Model file for the job. Use its own axes, mm. Face numbers are marked on the shaded views. Coordinates: 2 decimals unless noted, no trailing zeros. Write each loop counter-clockwise with the first axis right and the second up, starting at its lowest first coordinate (ties: lowest second). Pieces come first, ordered by that corner, then holes. Notation, with made-up numbers: (23.5, -12) - (75.5, -12) arc R23 ccw to (75.5, 11) - close; hole circle Ø5 at (41.25, 24). An arc over 180 degrees is marked (long way). Put each result on its own line as item: value. Start each with the question number.
1. Saw through at B-B, the plane z = -3.1. Write the cut outline in (x, y).
2. Drill centre lines: L1, parallel to Y at x = 686.5, z = -1.85; L2, parallel to Z at x = 697, y = -1297; L3, parallel to X at y = -1252, z = -1.25. Where is each one in solid material? Low to high. Write a range as from..to.
3. Drop flat-ended pins along their axis: P1, Ø2, axis at y = -1269.5, z = -2.5, coming from the +X side; P2, Ø4, axis at x = 681, y = -1314, coming from the -Z side. Give the stop position or say it passes through.
4. Saw through at A-A, the plane x = 663. Write the cut outline in (y, z).
5. Pull direction Y, two halves, no side cores. Call the marked faces 1 and 2: released by +Y, released by -Y, zero draft, split by the parting line, or undercut.
6. Saw through at C-C, the plane y = -1236. Write the cut outline in (x, z).
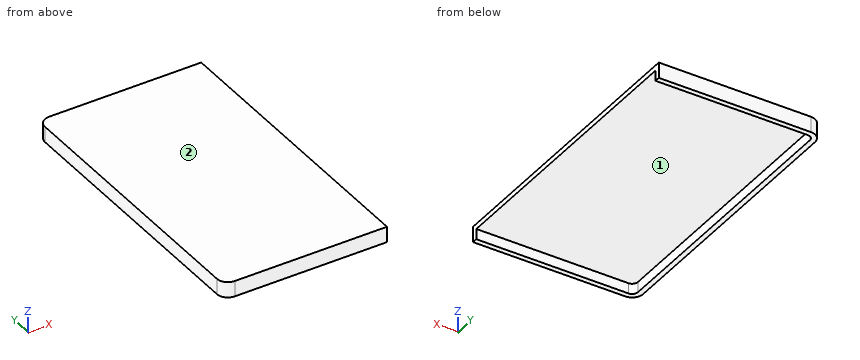
```python
from build123d import *

# Parameters (mm, degrees)
BOSS_EXTRUDE1_DEPTH = 2
BOSS_EXTRUDE2_START = -4
BOSS_EXTRUDE2_DEPTH = 4


with BuildPart() as part:
    # Sketch1 → Boss-Extrude1 (new body)
    with BuildSketch(Plane.XY):
        with BuildLine():
            ThreePointArc((661.511242052, -1226.030951231), (658.541393571, -1227.26110275), (657.311242052, -1230.230951231))
            Line((657.311242052, -1230.230951231), (657.311242052, -1334.010951231))
            ThreePointArc((657.311242052, -1334.010951231), (658.541393571, -1336.980799712), (661.511242052, -1338.210951231))
            Line((661.511242052, -1338.210951231), (719.851242052, -1338.210951231))
            Line((719.851242052, -1338.210951231), (719.851242052, -1336.210951231))
            Line((719.851242052, -1336.210951231), (661.511242052, -1336.210951231))
            ThreePointArc((661.511242052, -1336.210951231), (659.955607133, -1335.56658615), (659.311242052, -1334.010951231))
            Line((659.311242052, -1334.010951231), (659.311242052, -1230.230951231))
            ThreePointArc((659.311242052, -1230.230951231), (659.955607133, -1228.675316313), (661.511242052, -1228.030951231))
            Line((661.511242052, -1228.030951231), (719.851242052, -1228.030951231))
            Line((719.851242052, -1228.030951231), (719.851242052, -1226.030951231))
            Line((719.851242052, -1226.030951231), (661.511242052, -1226.030951231))
        make_face()
        with BuildLine():
            Line((719.851242052, -1261.620951231), (719.851242052, -1228.030951231))
            Line((719.851242052, -1228.030951231), (661.511242052, -1228.030951231))
            ThreePointArc((661.511242052, -1228.030951231), (659.955607133, -1228.675316313), (659.311242052, -1230.230951231))
            Line((659.311242052, -1230.230951231), (659.311242052, -1334.010951231))
            ThreePointArc((659.311242052, -1334.010951231), (659.955607133, -1335.56658615), (661.511242052, -1336.210951231))
            Line((661.511242052, -1336.210951231), (719.851242052, -1336.210951231))
            Line((719.851242052, -1336.210951231), (719.851242052, -1327.660951231))
            Line((719.851242052, -1327.660951231), (719.851242052, -1261.620951231))
        make_face()
    extrude(amount=BOSS_EXTRUDE1_DEPTH)

    # Sketch1_3 → Boss-Extrude2 (add)
    with BuildSketch(Plane.XY.offset(BOSS_EXTRUDE2_START)):
        with BuildLine():
            ThreePointArc((661.511242052, -1226.030951231), (658.541393571, -1227.26110275), (657.311242052, -1230.230951231))
            Line((657.311242052, -1230.230951231), (657.311242052, -1334.010951231))
            ThreePointArc((657.311242052, -1334.010951231), (658.541393571, -1336.980799712), (661.511242052, -1338.210951231))
            Line((661.511242052, -1338.210951231), (719.851242052, -1338.210951231))
            Line((719.851242052, -1338.210951231), (719.851242052, -1336.210951231))
            Line((719.851242052, -1336.210951231), (661.511242052, -1336.210951231))
            ThreePointArc((661.511242052, -1336.210951231), (659.955607133, -1335.56658615), (659.311242052, -1334.010951231))
            Line((659.311242052, -1334.010951231), (659.311242052, -1230.230951231))
            ThreePointArc((659.311242052, -1230.230951231), (659.955607133, -1228.675316313), (661.511242052, -1228.030951231))
            Line((661.511242052, -1228.030951231), (719.851242052, -1228.030951231))
            Line((719.851242052, -1228.030951231), (719.851242052, -1226.030951231))
            Line((719.851242052, -1226.030951231), (661.511242052, -1226.030951231))
        make_face()
    extrude(amount=BOSS_EXTRUDE2_DEPTH)


solid = part.part
```
Final values:
1. outline: (657.31, -1334.01) arc R4.2 ccw to (661.51, -1338.21) - (719.85, -1338.21) - (719.85, -1336.21) - (661.51, -1336.21) arc R2.2 cw to (659.31, -1334.01) - (659.31, -1230.23) arc R2.2 cw to (661.51, -1228.03) - (719.85, -1228.03) - (719.85, -1226.03) - (661.51, -1226.03) arc R4.2 ccw to (657.31, -1230.23) - close
2. L1: y = -1338.21..-1336.21, -1228.03..-1226.03
2. L2: z = 0..2
2. L3: x = 657.31..659.31
3. P1: stops at x = 659.31
3. P2: stops at z = 0
4. outline: (-1338.21, -4) - (-1336.21, -4) - (-1336.21, 0) - (-1228.03, 0) - (-1228.03, -4) - (-1226.03, -4) - (-1226.03, 2) - (-1338.21, 2) - close
5. face 1: undercut
5. face 2: zero draft
6. outline: (657.31, -4) - (659.31, -4) - (659.31, 0) - (719.85, 0) - (719.85, 2) - (657.31, 2) - close
